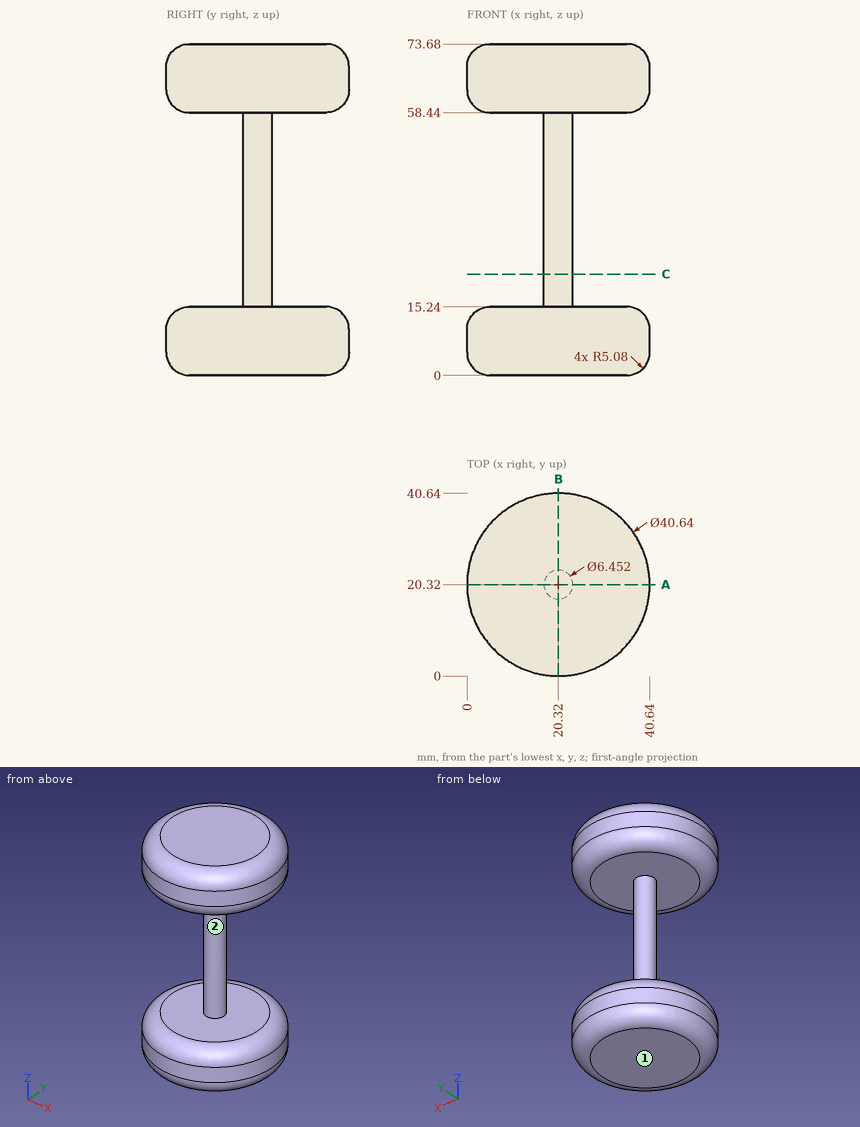
Geometry check sheet. Reference: drawing and pictorial views, mm from the part's lowest x, y, z. A direction names the side the tool comes from. Give positions to 0.01 mm unless a question says otherwise; leave off trailing zeros. Order: outer loops, then holes, each group sorted by start corner. A loop starts at its lowest first (then second) coordinate and runs counter-clockwise, first axis right, second up. Notation, with made-up numbers: (26.5, 17.5) - (64.5, 17.5) arc R15 ccw to (64.5, 29.5) - close; hole circle Ø9 at (-17.75, -27.5). An arc over 180 degrees is marked (long way). Answer as CSV lines item,"result". Start each with the question number.
Item 1: Material ranges on L1, parallel to Z at x = 27.5, y = 12.5; L2, parallel to Z at x = 27, y = 5; L3, parallel to Y at x = 23, z = 34 (1 decimal), recorded low to high.
Item 2: Access from +Z, -Z, +X, -X, +Y, -Y to the whole of each face (thin tool, end or side, straight path). Record for the marked faces 1 and 2.
Item 3: Section check C-C, the plane z = 22.5. Record the boundary of the cut face in (x, y), plus the area to 3 significant figures.
Item 4: Section check A-A, the plane y = 20.32. Record the boundary of the cut face in (x, z), plus the area to 3 significant figures.
Item 5: Gauge pin test, flat ends, axial feed: pin 1 (12 mm diameter, centred on y = 35.5, z = 25.5, fed in from +X); pin 2 (1 mm diameter, centred on y = 21, z = 40.5, fed in from -X); pin 3 (3 mm diameter, centred on y = 16.5, z = 39, fed in from +X). Record the tip position at first contact, or that the pin passes through.
Filled in:
1,L1,"0 to 15.24, 58.44 to 73.68"
1,L2,"0.22 to 15.02, 58.66 to 73.46"
1,L3,"18.5 to 22.1"
2,face 1,"-Z, +X, -X, +Y, -Y"
2,face 2,"none"
3,outline,"circle Ø6.45 at (20.32, 20.32)"
3,area,"32.7 mm^2"
4,outline,"(0, 5.08) arc R5.08 ccw to (5.08, 0) - (35.56, 0) arc R5.08 ccw to (40.64, 5.08) - (40.64, 10.16) arc R5.08 ccw to (35.56, 15.24) - (23.55, 15.24) - (23.55, 58.44) - (35.56, 58.44) arc R5.08 ccw to (40.64, 63.52) - (40.64, 68.6) arc R5.08 ccw to (35.56, 73.68) - (5.08, 73.68) arc R5.08 ccw to (0, 68.6) - (0, 63.52) arc R5.08 ccw to (5.08, 58.44) - (17.09, 58.44) - (17.09, 15.24) - (5.08, 15.24) arc R5.08 ccw to (0, 10.16) - close"
4,area,"1,470 mm^2"
5,pin 1,"through"
5,pin 2,"x = 17.1"
5,pin 3,"x = 22.56"
